Autodesk Inventor part; units mm, degrees
ref_plane "YZ Plane" through (0, 0, 0) normal (1, 0, 0) x (0, 1, 0)
ref_plane "XZ Plane" through (0, 0, 0) normal (0, 1, 0) x (-1, 0, 0)
ref_plane "XY Plane" through (0, 0, 0) normal (0, 0, 1) x (1, 0, 0)
sketch "Sketch1" plane through (0, 0, 0) normal (0, 1, 0) x (-1, 0, 0)
  arc A0 (0, -15) -> (0, 15) centre (-199.4367, 0) ccw
  line L0 (0, 15) -> (1, 15.0752)
  line L1 (0, -15) -> (1, -15.0752)
  arc A1 (1, -15.0752) -> (1, 15.0752) centre (-198.431, 0) ccw
  line L2 (1.5665, 1) -> (3.5665, 1)
  line L3 (3.5665, -1) -> (1.5665, -1)
  arc A2 (3.5665, -1) -> (3.5665, 1) centre (-196.431, 0) ccw
  point P0 (0, 0)
  point P1 (0.5633, 0)
  dimension "d0" = 200
  dimension "d1" = 30
  dimension "d2" = 1
  dimension "d3" = 1
  dimension "d4" = 200
  dimension "d5" = 1
  dimension "d6" = 1
  dimension "d7" = 2
  dimension "d8" = 2
  dimension "d9" = 200
extrude "Extrusion1" add sketch "Sketch1" along normal blind 20 contours A1 L2 A2 L3
extrude "Extrusion2" add sketch "Sketch1" along normal blind 10 contours A0 L0 A1 L1
ref_plane "Work Plane1" through (-3.5665, 20, 0) normal (0, 0, 1) x (1, 0, 0)
properties part number "silothingp2"
Verification items for the finished model (mm, model axes). A direction names the side the tool comes from. Coordinates: 2 decimals unless noted, no trailing zeros. Order: outer loops, then holes, each group sorted by start corner. A loop starts at its lowest first (then second) coordinate and runs counter-clockwise, first axis right, second up.
1. Sectioned sample at C-C, the plane z = 6. Record the cut outline in (x, y), and give its area (3 significant figures).
Results found:
outline: (-1.48, 0) - (-0.47, 0) - (-0.47, 10) - (-1.48, 10) - close
area: 10.1 mm2
2. Set-up check for faces 4 (the face through (-3, 10, 1)), 5 (the face through (-1, 0, 0)): record each of +Z, -Z, +X, -X, +Y, -Y from which the full face is reachable in a straight line by a thin tool's end or side.
Results found:
face 4: +Z, -X, +Y, -Y
face 5: +Z, -Z, +X, -X, -Y
3. Release check for a two-part mould opening along Z. For faces 1 (the face through (-3, 10, -1)), 2 (the face through (-1.403, 4.93, 8.141)), 3 (the face through (-0.563, 4.93, 0.21)) record: +Z half, -Z half, draft (parallel to the pull), parting line (faces both ways), or undercut.
Results found:
face 1: -Z half
face 2: +Z half
face 3: undercut
4. Go/stop test with flat-tipped pins: pin 1 Ø0.5 at (x, z) = (-0.5, 7.5) entering from +Y; pin 2 Ø1 at (x, y) = (-3, 11.5) entering from +Z; pin 3 Ø10 at (y, z) = (10.5, 7) entering from +X. Record where each tip stops, or that it passes through.
Results found:
pin 1: stops at y = 10
pin 2: stops at z = 1
pin 3: stops at x = -0.2
5. Sectioned sample at B-B, the plane x = -2.05. Record the cut outline in (y, z).
Results found:
outline: (0, -1) - (20, -1) - (20, 1) - (0, 1) - close
6. Sectioned sample at A-A, the plane y = 6.5. Record the cut outline in (x, z), and give its area (3 significant figures).
Results found:
outline: (-3.57, -1) - (-1.57, -1) arc R200 ccw to (-1, -15.08) - (0, -15) arc R200 cw to (0, 15) - (-1, 15.08) arc R200 ccw to (-1.57, 1) - (-3.57, 1) arc R200 ccw to start
area: 34.2 mm2
7. Scan lines: line 1 (Y direction, x = -0.5, z = 7.5); line 2 (Z direction, x = -2.75, y = 9.25); line 3 (X direction, y = 6.75, z = -0.5). Record each from-to range of solid material in increasing order.
Results found:
line 1: y = 0 to 10
line 2: z = -1 to 1
line 3: x = -3.57 to -0.56
